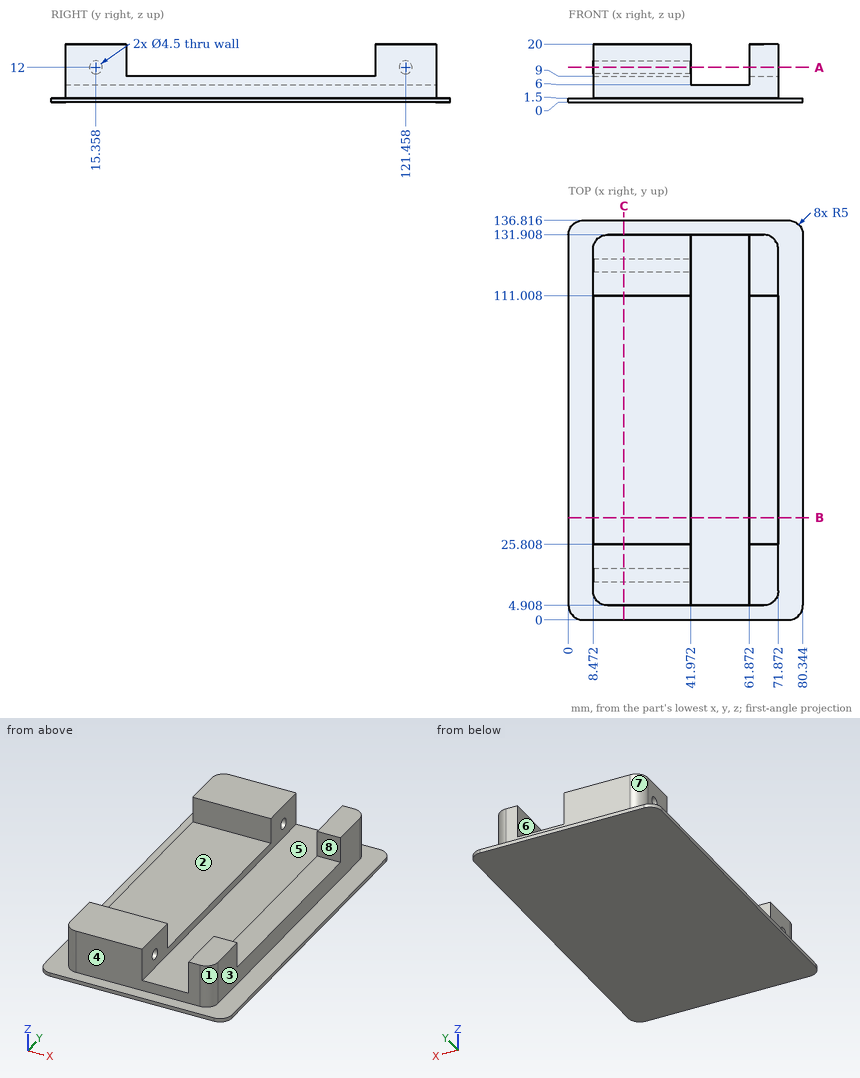
Can you work these out from the drawing? Everything is in mm from the part's minimum corner. A direction names the side the tool comes from. Give positions to 0.01 mm unless a question says otherwise; leave off trailing zeros. Order: outer loops, then holes, each group sorted by start corner. A loop starts at its lowest first (then second) coordinate and runs counter-clockwise, first axis right, second up. Notation, with made-up numbers: M -1,9.25 L 46,9.25 A18 cw 46,40.25 Z; hole C 23.25,67.25 d3. An arc over 180 degrees is marked long. Use a Markdown table: item, result. Add a question column.
Item 1: We'd pull the mould along X, two halves only. Please class the marked faces 6, 7 and 8: +X half, -X half, draft (parallel to the pull), parting line (faces both ways), or undercut.
Item 2: Will these pins go through, and if not, where does the flat tip stop? pin 1 (5 mm diameter, centred on y = 120.5, z = 6, fed in from -X); pin 2 (10 mm diameter, centred on x = 20.5, y = 63, fed in from +Z); pin 3 (3.5 mm diameter, centred on x = 27, z = 14.5, fed in from +Y).
Item 3: If I drill on L1, parallel to Y at x = 27.5, z = 12; L2, parallel to Y at x = 15, z = 16.5; L3, parallel to X at y = 55, z = 8.75, over which ranges is the centre line in solid material (lowest first)? Write a range as [from, to].
Item 4: For the marked faces 1, 2, 3, 4 and 5, which set-ups out of +Z, -Z, +X, -X, +Y, -Y let a thin tool reach every point of the face, with its end or its side?
Item 5: Suppose I cut it at B-B (y = 35). List the corners of the cut face in (x, z) for me, then the cut area to 3 significant figures.
Item 6: Suppose I cut it at A-A (z = 12). List the corners of the cut face in (x, y) for me.
Item 7: Suppose I cut it at C-C (x = 19). List the corners of the cut face in (y, z) for me.
Answer sheet:
| question | item | result |
|---|---|---|
| 1 | face 6 | undercut |
| 1 | face 7 | -X half |
| 1 | face 8 | draft |
| 2 | pin 1 | stops at x = 8.47 |
| 2 | pin 2 | stops at z = 9 |
| 2 | pin 3 | stops at y = 131.91 |
| 3 | L1 | y = [4.91, 13.11], [17.61, 25.81], [111.01, 119.21], [123.71, 131.91] |
| 3 | L2 | y = [4.91, 25.81], [111.01, 131.91] |
| 3 | L3 | x = [8.47, 41.97], [61.87, 71.87] |
| 4 | face 1 | +Z, +X, -Y |
| 4 | face 2 | +Z, +X, -X |
| 4 | face 3 | +Z, +X, +Y, -Y |
| 4 | face 4 | +Z, +X, -X, -Y |
| 4 | face 5 | +Z, +Y, -Y |
| 5 | outline | M 0,0 L 80.34,0 L 80.34,1.5 L 71.87,1.5 L 71.87,9 L 61.87,9 L 61.87,6 L 41.97,6 L 41.97,9 L 8.47,9 L 8.47,1.5 L 0,1.5 Z |
| 5 | area | 536 mm² |
| 6 | outline | M 8.47,9.91 A5 ccw 13.47,4.91 L 41.97,4.91 L 41.97,13.11 L 8.47,13.11 Z; M 8.47,17.61 L 41.97,17.61 L 41.97,25.81 L 8.47,25.81 Z; M 8.47,111.01 L 41.97,111.01 L 41.97,119.21 L 8.47,119.21 Z; M 8.47,123.71 L 41.97,123.71 L 41.97,131.91 L 13.47,131.91 A5 ccw 8.47,126.91 Z; M 61.87,4.91 L 66.87,4.91 A5 ccw 71.87,9.91 L 71.87,25.81 L 61.87,25.81 Z; M 61.87,111.01 L 71.87,111.01 L 71.87,126.91 A5 ccw 66.87,131.91 L 61.87,131.91 Z |
| 7 | outline | M 0,0 L 136.82,0 L 136.82,1.5 L 131.91,1.5 L 131.91,20 L 111.01,20 L 111.01,9 L 25.81,9 L 25.81,20 L 4.91,20 L 4.91,1.5 L 0,1.5 Z; hole C 15.36,12 d4.5; hole C 121.46,12 d4.5 |
